Design review of the part shown in the three views and the two pictorial views. Dimensions are in mm from the part's minimum x, y and z. Give positions to 0.01 mm unless a question says otherwise; leave off trailing zeros. Loops run counter-clockwise (first coordinate to the right, second up) from the corner with the lowest first, then second, coordinate; pieces in that order, holes last. Notation, with made-up numbers: (71, 4) - (129, 4) arc R18 ccw to (129, 26) - close; hole circle Ø3 at (13.5, 70.5). An arc over 180 degrees is marked (long way). Use CSV: the item, a comma, the result in double quotes. Start each with the question number.
1. Wall thickness on line 1 (X direction, y = 22, z = 3); line 2 (Z direction, x = 30, y = 3); line 3 (X direction, y = 22.25, z = 12.25): over which ranges is each line inside the solid? List them lowest first.
2. Take a section at C-C on x = 39. Give the boundary of the cut face in (y, z).
3. Take a section at B-B on x = 30. Give the boundary of the cut face in (y, z).
4. Take a section at A-A on y = 24.5. Give the boundary of the cut face in (x, z), plus the area to 3 significant figures.
5. Mouldability with a two-part tool opening along X and no side actions: class the marked faces 1, 2 and 3 as pulls with the +X half, pulls with the -X half, needs draft (parallel to the pull), parting line crosses it, or undercut.
6. For pin 1 (2 mm diameter, centred on x = 38.5, y = 17, fed in from -Z), flat-tipped, find the tip position at first contact; note if it passes through.
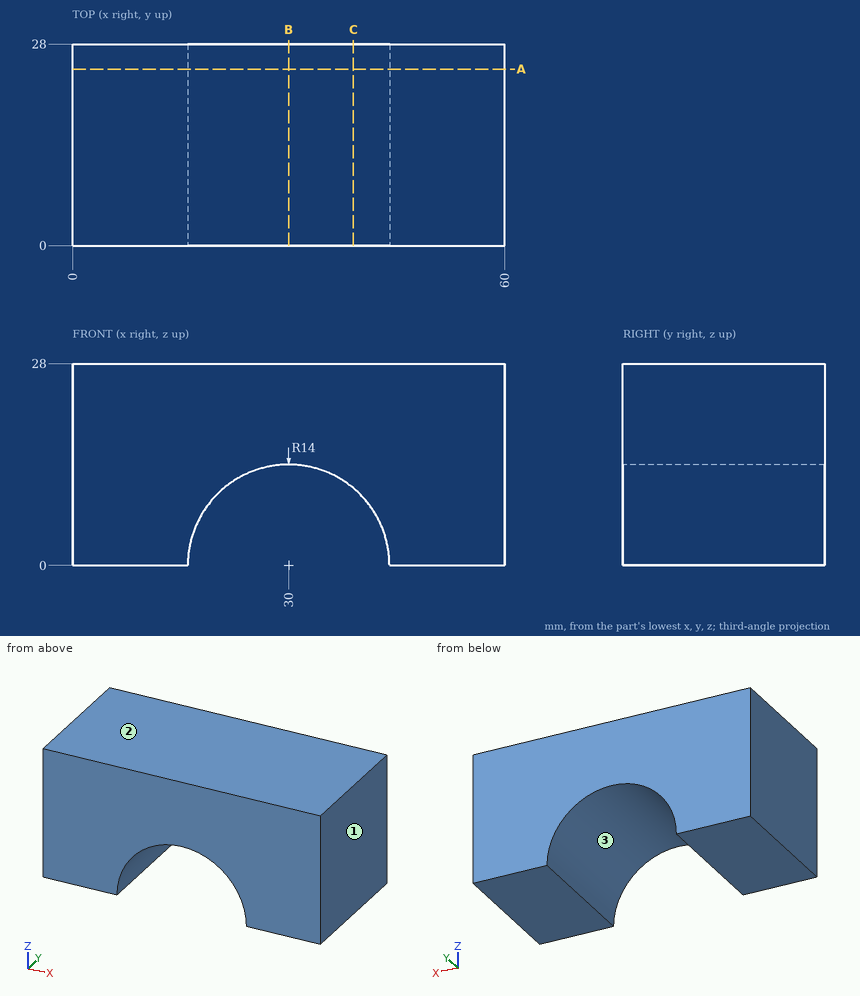
Check result:
1,line 1,"x = 0 to 16.33, 43.67 to 60"
1,line 2,"z = 14 to 28"
1,line 3,"x = 0 to 23.22, 36.78 to 60"
2,outline,"(0, 10.72) - (28, 10.72) - (28, 28) - (0, 28) - close"
3,outline,"(0, 14) - (28, 14) - (28, 28) - (0, 28) - close"
4,outline,"(0, 0) - (16, 0) arc R14 cw to (44, 0) - (60, 0) - (60, 28) - (0, 28) - close"
4,area,"1,370 mm²"
5,face 1,"pulls with the +X half"
5,face 2,"needs draft"
5,face 3,"undercut"
6,pin 1,"stops at z = 10.28"
